```python
from build123d import *

# Parameters (mm, degrees)
CUT_EXTRUDE_7_REACH              = 96.987
CUT_EXTRUDE_7_END_RADIUS         = 35
SKETCH_9_W                       = 22.863653518
SKETCH_9_H                       = 25.734556693
PATTERN_CIRCULAR_3_COUNT         = 8
SKETCH_11_W                      = 20
SKETCH_11_H                      = 7
EXTRUDE_1_DEPTH                  = 20
EXTRUDE_1_DIRECTION_2_REACH      = 96.987
EXTRUDE_1_DIRECTION_2_END_RADIUS = 40


with BuildPart() as part:
    # 草图1 → 旋转4 (revolve)
    with BuildSketch(Plane.XY, mode=Mode.PRIVATE) as revolve_4_sk:
        with BuildLine():
            Line((-35.764870687, -13.569622936), (-26.953430159, -24.560221363))
            Line((-26.953430159, -24.560221363), (-30.85448893, -27.687798773))
            Line((-30.85448893, -27.687798773), (-40, -16.2805108))
            Line((-40, -16.2805108), (-40, 30.977562367))
            ThreePointArc((-40, 30.977562367), (-39.707106781, 31.684669148), (-39, 31.977562367))
            Line((-39, 31.977562367), (-36, 31.977562367))
            ThreePointArc((-36, 31.977562367), (-35.292893219, 31.684669148), (-35, 30.977562367))
            Line((-35, 30.977562367), (-35, -3.569622936))
            Line((-35, -3.569622936), (-15.764870687, -3.569622936))
            Line((-15.764870687, -3.569622936), (-15.764870687, -13.569622936))
            Line((-15.764870687, -13.569622936), (-35.764870687, -13.569622936))
        make_face()
    revolve(revolve_4_sk.sketch.rotate(Axis((0, 0, 0), (0, 1, 0)), 270), axis=Axis((0, 0, 0), (0, 1, 0)))

    # 切除-拉伸7: up to this cylinder (the profile starts outside it)
    cut_extrude_7_end = Plane(origin=(0, 14.581038, 0), z_dir=(0, -1, 0)) * Cylinder(CUT_EXTRUDE_7_END_RADIUS, 264.974, mode=Mode.PRIVATE)
    # 草图9 → 切除-拉伸7 (cut, up to the surface)
    with BuildSketch(Plane.XY.offset(40), mode=Mode.PRIVATE) as cut_extrude_7_sk1:
        with Locations((0, 14.581037932)):
            Rectangle(SKETCH_9_W, SKETCH_9_H)
    cut_extrude_7_tool1 = extrude(cut_extrude_7_sk1.sketch, amount=-CUT_EXTRUDE_7_REACH, mode=Mode.PRIVATE) - cut_extrude_7_end
    cut_extrude_7 = cut_extrude_7_tool1.solids().sort_by_distance((0, 14.581038, 40))[0]
    add(cut_extrude_7, mode=Mode.SUBTRACT)

    # 阵列(圆周)3: 切除-拉伸7 ×8 about axis
    pattern_circular_3_axis = Axis((0, 0, 0), (0, 1, 0))
    for i in range(1, PATTERN_CIRCULAR_3_COUNT):
        add(cut_extrude_7.rotate(pattern_circular_3_axis, i * 360 / PATTERN_CIRCULAR_3_COUNT), mode=Mode.SUBTRACT)

    # 草图11 → 凸台-拉伸1 (add)
    with BuildSketch(Plane.XY.offset(40)):
        with Locations((0, -6.301485772)):
            Rectangle(SKETCH_11_W, SKETCH_11_H)
    extrude(amount=EXTRUDE_1_DEPTH)

    # 凸台-拉伸1 direction 2: up to this cylinder (the profile starts outside it)
    extrude_1_direction_2_end = Plane(origin=(0, -6.301486, 0), z_dir=(0, -1, 0)) * Cylinder(EXTRUDE_1_DIRECTION_2_END_RADIUS, 274.974, mode=Mode.PRIVATE)
    # 草图11 → 凸台-拉伸1 direction 2 (add, up to the surface)
    with BuildSketch(Plane.XY.offset(40), mode=Mode.PRIVATE) as extrude_1_direction_2_sk1:
        with Locations((0, -6.301485772)):
            Rectangle(SKETCH_11_W, SKETCH_11_H)
    extrude_1_direction_2_tool1 = extrude(extrude_1_direction_2_sk1.sketch, amount=-EXTRUDE_1_DIRECTION_2_REACH, mode=Mode.PRIVATE) - extrude_1_direction_2_end
    add(extrude_1_direction_2_tool1.solids().sort_by_distance((0, -6.301486, 40))[0])
    add(extrude_1_direction_2_tool1.solids().sort_by_distance((0, -6.301486, 40))[1])


solid = part.part
```
Geometry check sheet. Reference: the model listing, model coordinates, mm. A direction names the side the tool comes from. Round coordinates to 2 decimals unless told otherwise and drop trailing zeros. Write each loop counter-clockwise with the first axis right and the second up, starting at its lowest first coordinate (ties: lowest second). Pieces come first, ordered by that corner, then holes. Notation, with made-up numbers: (87.25, -4.5) - (146.25, -4.5) arc R4 ccw to (146.25, -0.5) - close; hole circle Ø2 at (35, 24.5). An arc over 180 degrees is marked (long way). Write each question's results on one line, items separated by ' | '.
(1) Depth check by flat-ended pin: pin 1 Ø8 at (x, z) = (13, -8) entering from -Y; pin 2 Ø5 at (y, z) = (-10.5, 3) entering from -X; pin 3 Ø10 at (x, z) = (20.5, -29.5) entering from -Y. Enter the tip coordinate at first touch or a pass-through.
Computed:
pin 1: stops at y = -13.57 | pin 2: stops at x = -40 | pin 3: stops at y = -27.6
(2) Thickness scan on probe 1 along X at (y, z) = (-9.5, 0); probe 2 along Y at (x, z) = (-2, 26.5); probe 3 along Y at (x, z) = (3, 42). Record the ranges inside material, lowest first. Write a range as from..to.
Computed:
probe 1: x = -40..-15.76, 15.76..40 | probe 2: y = -13.57..-3.57 | probe 3: y = -9.8..-2.8
(3) Set-up check for faces 4 (the face through (33.357, 14.401, -17.19)), 5 (the face through (11.432, 14, 36)), 6 (the face through (34.5, 31.978, -11.4)), 7 (the face through (36, 14, -11.432)), 8 (the face through (-8.225, -24.027, -26.117)): record each of +Z, -Z, +X, -X, +Y, -Y from which the full face is reachable in a straight line by a thin tool's end or side.
Computed:
face 4: -Z | face 5: +Z, -Z | face 6: +Z, -Z, +X, -X, +Y | face 7: +X, -X | face 8: none
(4) Draft check along Y on faces 1 (the face through (15, -3.57, -7)), 2 (the face through (26, 27.448, -26)), 3 (the face through (10, -6, 50)). Enter one of: pulls with the +Y half, pulls with the -Y half, needs draft (parallel to the pull), parting line crosses it, or undercut.
Computed:
face 1: pulls with the +Y half | face 2: undercut | face 3: needs draft
(5) Sectioned sample at A-A, the plane y = 24. Count the separate pieces of the cut face and the enclosed holes in it, plus the area to 3 significant figures.
Computed:
separate pieces: 8 | enclosed holes: 0 | area: 249 mm^2
(6) Sectioned sample at D-D, the plane y = -7.5. Enter the section's corners in (x, z), plus the area to 3 significant figures.
Computed:
outline: (-10, 38.73) arc R40 ccw (long way) to (10, 38.73) - (10, 60) - (-10, 60) - close; hole circle Ø31.53 at (0, 0) | area: 4,650 mm^2
